from build123d import *

# Parameters (mm, degrees)
F0_R          = 1.6
F1_DEPTH      = 16
F1_DEPTH_BACK = 9
F3_R          = 3.5
F3_R_2        = 1.4
F4_DEPTH      = 22
F5_DEPTH      = 16.501
F8_R          = 9.65
F9_DEPTH      = 5
F10_R         = 4.25
F11_DEPTH     = 6.5
F12_W         = 25
F12_H         = 9.1
F13_DEPTH     = 6.6
F14_R         = 2.8
F15_DEPTH     = 3
F16_W         = 8
F16_H         = 6
F16_H_2       = 9.1
F17_DEPTH     = 11
F23_W         = 8
F23_H         = 14.5
F24_DEPTH     = 25.001
F25_W         = 14
F25_H         = 9.5
F26_DEPTH     = 14.5
F28_DEPTH     = 9.0010001359
F29_W         = 14
F29_H         = 4
F30_DEPTH     = 6
F32_DEPTH     = 2.4
F33_W         = 10
F33_H         = 14.5
F34_DEPTH     = 4
F35_R         = 0.9
F36_DEPTH     = 3.2
F37_W         = 8.5
F37_H         = 12
F38_DEPTH     = 5
F39_R         = 0.9
F40_DEPTH     = 12
F41_SIZE      = 0.25
F42_T1_DEPTH  = 31.0668298797
F42_T3_DEPTH  = 28.5668298797


# Not quite as in the source:
# - a fillet or chamfer that OpenCascade refuses, or shapes differently, is made with other operations: its cross-section is extruded or revolved along the edge and cut away or added


with BuildPart() as f1:
    # F0 (on Right) → F1 (new body, two sides)
    with BuildSketch(Plane.YZ) as f1_sk:
        Polygon((-12.5, 0), (15, 0), (15, 38.5), (-10, 38.5), (-10, 24), (-12.5, 24), align=None)
        with Locations((-9.5, 9.5)):
            Circle(F0_R, mode=Mode.SUBTRACT)
        with Locations((9.5, 9.5)):
            Circle(F0_R, mode=Mode.SUBTRACT)
    extrude(amount=F1_DEPTH)
    extrude(f1_sk.sketch, amount=-F1_DEPTH_BACK)

    # F3 (on face) → F4 (cut)
    with BuildSketch(Plane(origin=(0, 0, 0), x_dir=(1, 0, 0), z_dir=(0, 0, -1))):
        Circle(F3_R)
        with Locations((-2.2609790798, 6.2119889676)):
            Circle(F3_R_2)
        with Locations((-4.2492507141, -5.0640598044)):
            Circle(F3_R_2)
        with Locations((6.5102297939, -1.1479291633)):
            Circle(F3_R_2)
    extrude(amount=-F4_DEPTH, mode=Mode.SUBTRACT)

    # F5 (cut, through all): a face of the model
    f5_faces = [f1.faces().sort_by_distance(p)[0] for p in [
        (0, 0, 22),
    ]]
    extrude(f5_faces, amount=-F5_DEPTH, mode=Mode.SUBTRACT)

    # F8 (on face) → F9 (cut)
    with BuildSketch(Plane(origin=(0, 0, 0), x_dir=(1, 0, 0), z_dir=(0, 0, -1))):
        Circle(F8_R)
    extrude(amount=-F9_DEPTH, mode=Mode.SUBTRACT)

    # F10 (on face) → F11 (cut)
    with BuildSketch(Plane(origin=(0, 0, 5), x_dir=(1, 0, 0), z_dir=(0, 0, -1))):
        Circle(F10_R)
    extrude(amount=-F11_DEPTH, mode=Mode.SUBTRACT)

    # F12 (on face) → F13 (cut)
    with BuildSketch(Plane.YZ.offset(16)):
        with Locations((2.5, 28.55)):
            Rectangle(F12_W, F12_H)
    extrude(amount=-F13_DEPTH, mode=Mode.SUBTRACT)

    # F14 (on face) → F15 (cut)
    with BuildSketch(Plane(origin=(-9, 0, 0), x_dir=(0, -1, 0), z_dir=(-1, 0, 0))):
        with Locations((-9.5, 9.5)):
            Circle(F14_R)
        with BuildLine():
            ThreePointArc((9.5, 6.7), (11.4798989873, 7.5201010127), (12.3, 9.5))
            ThreePointArc((12.3, 9.5), (11.4798989873, 11.4798989873), (9.5, 12.3))
            ThreePointArc((9.5, 12.3), (6.7, 9.5), (9.5, 6.7))
        make_face()
        with BuildLine():
            ThreePointArc((9.5, 12.3), (11.4798989873, 11.4798989873), (12.3, 9.5))
            ThreePointArc((12.3, 9.5), (11.4798989873, 7.5201010127), (9.5, 6.7))
            Line((9.5, 6.7), (12.5, 6.7))
            Line((12.5, 6.7), (12.5, 12.3))
            Line((12.5, 12.3), (9.5, 12.3))
        make_face()
    extrude(amount=-F15_DEPTH, mode=Mode.SUBTRACT)

    # F16 (on face) → F17 (cut)
    with BuildSketch(Plane.YZ.offset(16)):
        with Locations((-8.5, 21)):
            Rectangle(F16_W, F16_H)
        with Locations((-8.5, 28.55)):
            Rectangle(F16_W, F16_H_2)
    extrude(amount=-F17_DEPTH, mode=Mode.SUBTRACT)

    # F21 (on plane+point) → F22 (revolve, cut)
    with BuildSketch(Plane.XZ.offset(-11)):
        Polygon((0, 12.5), (0, 38.5), (-2.75, 38.5), (-2.75, 31.8), (-1.4, 31.8), (-1.4, 12.5), align=None)
    revolve(axis=Axis((0, 11, 25.5), (0, 0, 1)), mode=Mode.SUBTRACT)

    # F23 (on face) → F24 (cut, through all)
    with BuildSketch(Plane.YZ.offset(16)):
        with Locations((-8.5, 31.25)):
            Rectangle(F23_W, F23_H)
    extrude(amount=-F24_DEPTH, mode=Mode.SUBTRACT)

    # F25 (on face) → F26 (cut, through all)
    with BuildSketch(Plane.XY.offset(38.5)):
        with Locations((-2, 0.25)):
            Rectangle(F25_W, F25_H)
    extrude(amount=-F26_DEPTH, mode=Mode.SUBTRACT)

    # F27 (on face) → F28 (cut, through all)
    with BuildSketch(Plane(origin=(-9, 0, 0), x_dir=(0, -1, 0), z_dir=(-1, 0, 0))):
        with BuildLine():
            Line((-9.65, 0), (9.65, 0))
            ThreePointArc((9.65, 0), (7.4518594557, 3.5930041952), (3.4817380717, 5))
            Line((3.4817380717, 5), (-3.4817380717, 5))
            ThreePointArc((-3.4817380717, 5), (-7.4518594557, 3.5930041952), (-9.65, 0))
        make_face()
    extrude(amount=-F28_DEPTH, mode=Mode.SUBTRACT)

    # F29 (on face) → F30 (cut, through all)
    with BuildSketch(Plane.XY.offset(24)):
        with Locations((-2, -10.5)):
            Rectangle(F29_W, F29_H)
    extrude(amount=-F30_DEPTH, mode=Mode.SUBTRACT)

    # F31 (on face) → F32 (join)
    with BuildSketch(Plane(origin=(0, 15, 0), x_dir=(-1, 0, 0), z_dir=(0, 1, 0))):
        Polygon((-23.2, 0), (-16, 0), (-16, 24), (-16.1, 24), (-16.1, 33.1), (-16, 33.1), (-16, 38.5), (-23.2, 38.5), align=None)
    extrude(amount=-F32_DEPTH)

    # F33 (on face) → F34 (cut)
    with BuildSketch(Plane(origin=(-9, 0, 0), x_dir=(0, -1, 0), z_dir=(-1, 0, 0))):
        with Locations((-10, 31.25)):
            Rectangle(F33_W, F33_H)
    extrude(amount=-F34_DEPTH, mode=Mode.SUBTRACT)

    # F35 (on face) → F36 (cut)
    with BuildSketch(Plane(origin=(-5, 0, 0), x_dir=(0, -1, 0), z_dir=(-1, 0, 0))):
        with Locations((-10, 33.75)):
            Circle(F35_R)
        with Locations((-10, 27.25)):
            Circle(F35_R)
    extrude(amount=-F36_DEPTH, mode=Mode.SUBTRACT)

    # F37 (on face) → F38 (join)
    with BuildSketch(Plane(origin=(0, 15, 0), x_dir=(-1, 0, 0), z_dir=(0, 1, 0))):
        with Locations((-27.45, 6)):
            Rectangle(F37_W, F37_H)
    extrude(amount=-F38_DEPTH)

    # F39 (on face) → F40 (cut, through all)
    with BuildSketch(Plane.XY.offset(12)):
        with Locations((27.45, 12.55)):
            Circle(F39_R)
    extrude(amount=-F40_DEPTH, mode=Mode.SUBTRACT)

    # F41
    f41_edges = [f1.edges().sort_by_distance(p)[0] for p in [
        (-3.660979, -6.211989, 5),
        (5.11023, 1.147929, 5),
        (-5.649251, 5.06406, 5),
    ]]
    chamfer(f41_edges, length=F41_SIZE)

    # F42: chamfer of 5 on 2 edges, made by hand

    # F42_s2 → F42_t1 (cut)
    with BuildSketch(Plane.XZ.offset(-27.8584149398)):
        Polygon((-9, 5), (-4, 0), (-9, 0), align=None)
    extrude(amount=F42_T1_DEPTH, mode=Mode.SUBTRACT)

    # F42_s4 → F42_t3 (cut)
    with BuildSketch(Plane.XZ.offset(-3.2084149398)):
        Polygon((-9, 5), (-4, 0), (-9, 0), align=None)
    extrude(amount=F42_T3_DEPTH, mode=Mode.SUBTRACT)


solid = f1.part
Can you work these out from the model? Positions are in its coordinate system, mm. A direction names the side the tool comes from. Coordinates: 2 decimals unless noted, no trailing zeros. Order: outer loops, then holes, each group sorted by start corner. A loop starts at its lowest first (then second) coordinate and runs counter-clockwise, first axis right, second up. Notation, with made-up numbers: (-2, -2) - (43, -2) arc R24 ccw to (43, 18) - close; hole circle Ø1 at (5, -2). An arc over 180 degrees is marked (long way). Answer as a JSON object with one key per item and string values. Group by question number.
Q1. We'd pull the mould along Y, two halves only. Please class faces 1 (the face through (-5.19, -8.56, 2.43)), 2 (the face through (28.5, 12.5, 12)), 3 (the face through (-2, -8.5, 21)): +Y half, -Y half, draft (parallel to the pull), parting line (faces both ways), or undercut.
Q2. On a 3-axis mill with a long thin cutter (end or side, diameter ignored), from which of +Z, -Z, +X, -X, +Y, -Y can I reach the whole of each face in a straight line? I mean faces 4 (the face through (5.11, 1.09, 13.51)), 5 (the face through (-8, -11, 12.3)), 6 (the face through (0, 11, 12.5)), 7 (the face through (-7.52, 6.83, 10.34)). Say none if no direction works.
Q3. I need wall thicknesses on line 1 (Y direction, x = -4.2, z = 33.75); line 2 (Y direction, x = 0, z = 30.5); line 3 (Z direction, x = 3, y = -9.5). Which ranges of each line are inside material? Lowest first, please. Write a range as from..to.
Q4. Imagine slicing it at D-D (y = -10.5). Please give me the cut outline in (x, z).
Q5. Imagine slicing it at B-B (z = 27.25). Please give me the cut outline in (x, y), and give its area (3 significant figures).
Q6. Imagine slicing it at A-A (x = 12.5). Please give me the cut outline in (y, z), and give its area (3 significant figures).
Q7. Imagine slicing it at C-C (z = 9.5). Please give me the cut outline in (x, y), and give its area (3 significant figures).
Q8. Will these pins go through, and if not, where does the flat tip stop? P1, Ø1.4, axis at x = 27.45, y = 12.55, coming from the -Z side; P2, Ø3, axis at y = 9.5, z = 14.5, coming from the +X side; P3, Ø1.7, axis at x = -2.26, y = -6.21, coming from the -Z side; P4, Ø12, axis at x = 11.5, z = 25.5, coming from the -Y side.
Determined:
{
 "1": {"face 1": "undercut", "face 2": "draft", "face 3": "-Y half"},
 "2": {"face 4": "-Z", "face 5": "-X, -Y", "face 6": "+Z", "face 7": "-X"},
 "3": {"line 1": "y = 5..9.1, 10.9..15", "line 2": "y = 5..9.6, 12.4..15", "line 3": "z = 0..7.9, 11.1..18"},
 "4": {"outline": "(-9, 5) - (-4, 0) - (16, 0) - (16, 8.25) - (-6, 8.25) - (-6, 6.7) - (-9, 6.7) - close; (-9, 12.3) - (-6, 12.3) - (-6, 10.75) - (16, 10.75) - (16, 18) - (-9, 18) - close"},
 "5": {"outline": "(-5, 5) - (5, 5) - (5, -4.5) - (9.4, -4.5) - (9.4, 15) - (-5, 15) - (-5, 10.9) - (-1.8, 10.9) - (-1.8, 9.1) - (-5, 9.1) - close; (16.1, 12.6) - (23.2, 12.6) - (23.2, 15) - (16.1, 15) - close; hole circle Ø2.8 at (0, 11)", "area": "191 mm2"},
 "6": {"outline": "(-12.5, 0) - (15, 0) - (15, 24) - (-4.5, 24) - (-4.5, 18) - (-12.5, 18) - close; (-4.5, 33.1) - (15, 33.1) - (15, 38.5) - (-4.5, 38.5) - close; hole circle Ø3.2 at (-9.5, 9.5); hole circle Ø3.2 at (9.5, 9.5)", "area": "701 mm2"},
 "7": {"outline": "(-9, -6.7) - (-6, -6.7) - (-6, -7.9) - (16, -7.9) - (16, 7.9) - (-6, 7.9) - (-6, 6.7) - (-9, 6.7) - close; (-9, 12.3) - (-6, 12.3) - (-6, 11.1) - (16, 11.1) - (16, 12.6) - (23.2, 12.6) - (23.2, 10) - (31.7, 10) - (31.7, 15) - (-9, 15) - close; (-6, -12.5) - (16, -12.5) - (16, -11.1) - (-6, -11.1) - close; hole circle Ø2.8 at (-4.25, 5.06); hole circle Ø8.5 at (0, 0); hole circle Ø2.8 at (-2.26, -6.21); hole circle Ø2.8 at (6.51, 1.15); hole circle Ø1.8 at (27.45, 12.55)", "area": "495 mm2"},
 "8": {"P1": "passes through", "P2": "stops at x = 16", "P3": "stops at z = 22", "P4": "stops at y = -4.5"}
}
